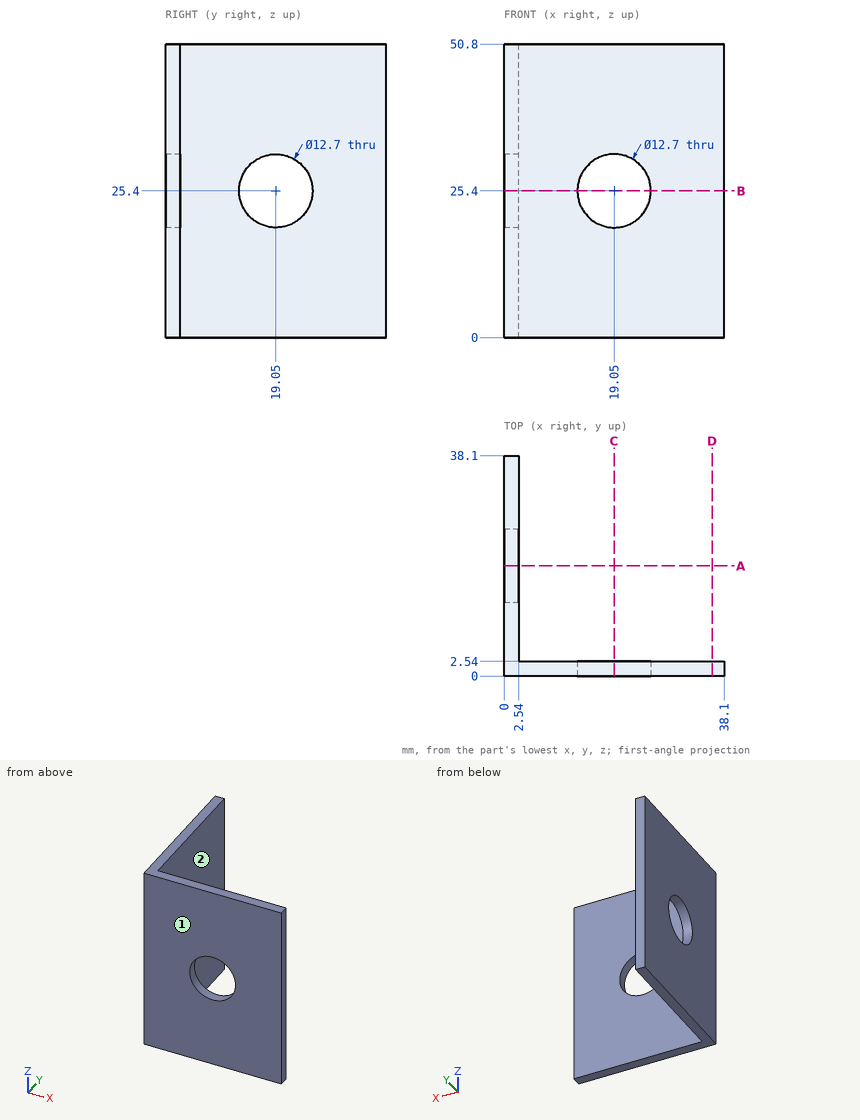
Print and shaded views of the part. All mm, measured from the part's lowest x, y and z. A direction names the side the tool comes from. Give positions to 0.01 mm unless a question says otherwise; leave off trailing zeros. Write each loop counter-clockwise with the first axis right and the second up, starting at its lowest first coordinate (ties: lowest second). Pieces come first, ordered by that corner, then holes. Notation, with made-up numbers: (58.5, 86.5) -> (69.5, 86.5) arc R15 ccw to (69.5, 94.5) -> close; hole circle Ø7 at (74, 41). An arc over 180 degrees is marked (long way). Write each question's results on one line, items separated by ' | '.
1. Cut at A-A, the plane y = 19.05. Write the cut outline in (x, z), then the cut area to 3 significant figures.
Geometry check:
outline: (0, 0) -> (2.54, 0) -> (2.54, 19.05) -> (0, 19.05) -> close; (0, 31.75) -> (2.54, 31.75) -> (2.54, 50.8) -> (0, 50.8) -> close | area: 96.8 mm²
2. Cut at B-B, the plane z = 25.4. Write the cut outline in (x, y).
Geometry check:
outline: (0, 0) -> (12.7, 0) -> (12.7, 2.54) -> (2.54, 2.54) -> (2.54, 12.7) -> (0, 12.7) -> close; (0, 25.4) -> (2.54, 25.4) -> (2.54, 38.1) -> (0, 38.1) -> close; (25.4, 0) -> (38.1, 0) -> (38.1, 2.54) -> (25.4, 2.54) -> close
3. Wall check: probe 1 along Z at (x, y) = (19.05, 0.85); probe 2 along X at (y, z) = (0.7, 25.4); probe 3 along Y at (x, z) = (1, 25). Give the ranges that are in metal, low to high. Write a range as [from, to].
Geometry check:
probe 1: [0, 19.05], [31.75, 50.8] | probe 2: [0, 12.7], [25.4, 38.1] | probe 3: [0, 12.71], [25.39, 38.1]
4. Which spindle directions (+Z, -Z, +X, -X, +Y, -Y) get a long thin tool onto all of the face, cutting with end or side? Do the marked faces 1 and 2. Say none if no direction does.
Geometry check:
face 1: +Z, -Z, +X, -X, -Y | face 2: +Z, -Z, +X, +Y
5. Drop a flat-ended pin along its axis: P1, Ø10, axis at x = 30.5, z = 14.5, coming from the +Y side. Give the stop position or say it passes through.
Geometry check:
P1: y = 2.54
6. Cut at D-D, the plane x = 36. Write the cut outline in (y, z).
Geometry check:
outline: (0, 0) -> (2.54, 0) -> (2.54, 50.8) -> (0, 50.8) -> close
